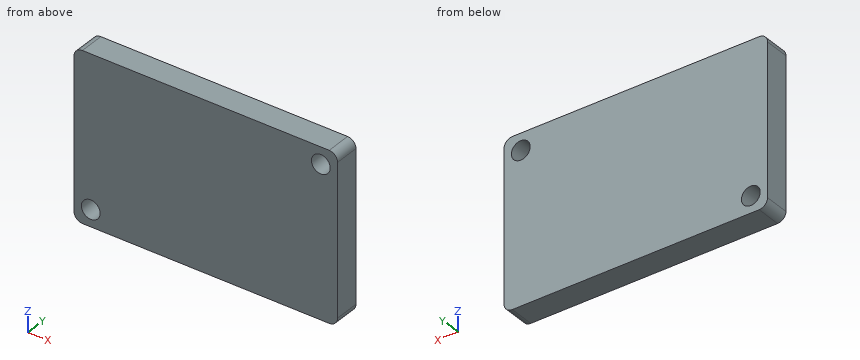
from build123d import *

# Parameters (mm, degrees)
SKETCH_1_W          = 63
SKETCH_1_H          = 6
BLOCKEXTRUDE_DEPTH  = 40
FILLET_2_R          = 2
SKETCH_2_R          = 2.25
MOUNTING_HOLE_DEPTH = 75.866547937
SKETCH_3_R          = 2.25
CUT_EXTRUDE_2_DEPTH = 75.866547937


with BuildPart() as part:
    # 草图1 → BlockExtrude (new body)
    with BuildSketch(Plane.XY):
        with Locations((31.5, 3)):
            Rectangle(SKETCH_1_W, SKETCH_1_H)
    extrude(amount=BLOCKEXTRUDE_DEPTH)

    # Fillet 2
    fillet_2_edges = [part.edges().sort_by_distance(p)[0] for p in [
        (63, 3, 40),
        (0, 3, 40),
        (63, 3, 0),
        (0, 3, 0),
    ]]
    fillet(fillet_2_edges, radius=FILLET_2_R)

    # 草图2 → Mounting_hole (cut, through all)
    with BuildSketch(Plane(origin=(0, 6, 0), x_dir=(1, 0, 0), z_dir=(0, 1, 0))):
        with Locations(Location((4, -4, 0), (0, 0, 270))):
            Circle(SKETCH_2_R)
    extrude(amount=-MOUNTING_HOLE_DEPTH, mode=Mode.SUBTRACT)

    # 草图3 → 切除-拉伸2 (cut, through all)
    with BuildSketch(Plane(origin=(0, 6, 0), x_dir=(1, 0, 0), z_dir=(0, 1, 0))):
        with Locations(Location((59, -36, 0), (0, 0, 270))):
            Circle(SKETCH_3_R)
    extrude(amount=-CUT_EXTRUDE_2_DEPTH, mode=Mode.SUBTRACT)


solid = part.part
Geometry check sheet. Reference: the model listing, model coordinates, mm. Round coordinates to 2 decimals unless told otherwise and drop trailing zeros. Order: outer loops, then holes, each group sorted by start corner. A loop starts at its lowest first (then second) coordinate and runs counter-clockwise, first axis right, second up. Notation, with made-up numbers: (80, 85) -> (85, 85) arc R17 ccw to (85, 103) -> close; hole circle Ø3 at (-10, 8.5). An arc over 180 degrees is marked (long way). Use one line per item in the form item = value.
1. Go/stop test with a flat-tipped pin: pin 1 (3.5 mm diameter, centred on x = 59, z = 36, fed in from +Y). Record where the tip stops, or that it passes through.
Working result:
pin_1 = through
2. Scan lines: line 1 along X through (y, z) = (3.5, 36); line 2 along X through (y, z) = (3.55, 4); line 3 along Z through (x, y) = (5.5, 4.4). Record each from-to range of solid material in increasing order. Write a range as from..to.
Working result:
line_1 = 0..56.75, 61.25..63
line_2 = 0..1.75, 6.25..63
line_3 = 0..2.32, 5.68..40
3. Cross-section at B-B, the plane x = 59. Enter the section's corners in (y, z), plus the area to 3 significant figures.
Working result:
outline = (0, 0) -> (6, 0) -> (6, 33.75) -> (0, 33.75) -> close; (0, 38.25) -> (6, 38.25) -> (6, 40) -> (0, 40) -> close
area = 213 mm^2
4. Cross-section at A-A, the plane z = 36. Enter the section's corners in (x, y), plus the area to 3 significant figures.
Working result:
outline = (0, 0) -> (56.75, 0) -> (56.75, 6) -> (0, 6) -> close; (61.25, 0) -> (63, 0) -> (63, 6) -> (61.25, 6) -> close
area = 351 mm^2
